Autodesk Inventor part; units mm, degrees
ref_plane "YZ Plane" through (0, 0, 0) normal (1, 0, 0) x (0, 1, 0)
ref_plane "XZ Plane" through (0, 0, 0) normal (0, 1, 0) x (-1, 0, 0)
ref_plane "XY Plane" through (0, 0, 0) normal (0, 0, 1) x (1, 0, 0)
sketch "Sketch1" plane through (0, 0, 0) normal (0, 1, 0) x (-1, 0, 0)
  circle A0 centre (0, 0) radius 30.734
  line L0 (-20.32, 68.58) -> (350.52, 68.58)
  line L1 (381, 38.1) -> (381, -38.1)
  line L2 (350.52, -68.58) -> (-20.32, -68.58)
  line L3 (-50.8, -38.1) -> (-50.8, 38.1)
  arc A1 (-20.32, 68.58) -> (-50.8, 38.1) centre (-20.32, 38.1) ccw
  arc A2 (-50.8, -38.1) -> (-20.32, -68.58) centre (-20.32, -38.1) ccw
  arc A3 (381, 38.1) -> (350.52, 68.58) centre (350.52, 38.1) ccw
  arc A4 (350.52, -68.58) -> (381, -38.1) centre (350.52, -38.1) ccw
  point P0 (-50.8, 68.58)
  point P1 (381, -68.58)
  point P2 (-50.8, -68.58)
  dimension "d0" = 61.468
  dimension "d1" = 137.16
  dimension "d2" = 431.8
  dimension "d3" = 50.8
  dimension "d4" = 68.58
  dimension "d5" = 30.48
extrude "Extrusion1" add sketch "Sketch1" against normal blind 129.54
sketch "Sketch2" plane through (0, -129.54, 0) normal (0, -1, 0) x (1, 0, 0)
  circle A0 centre (0, 0) radius 38.1
  dimension "d17" = 76.2
extrude "Extrusion2" add sketch "Sketch2" against normal blind 93.98
sketch "Sketch3" plane through (0, 0, 0) normal (0, 1, 0) x (1, 0, 0)
  line L0 (50.8, 38.1) -> (50.8, -38.1)
  line L1 (50.8, 0) -> (-132.08, 0)
  line L2 (20.32, -68.58) -> (-350.52, -68.58)
  line L3 (-132.08, -68.58) -> (-434.975, -68.58)
  line L4 (-434.975, -68.58) -> (-434.975, 68.58)
  line L5 (-434.975, 68.58) -> (-132.08, 68.58)
  line L6 (-132.08, 68.58) -> (-132.08, -68.58)
  point P0 (0, 0)
  dimension "d10" = 182.88
extrude "Extrusion3" cut sketch "Sketch3" against normal blind 35.2425
sketch "Sketch4" plane through (0, -35.2425, 0) normal (0, 1, 0) x (1, 0, 0)
  line L0 (-381, -38.1) -> (-381, 38.1)
  line L1 (-381, 0) -> (-328.6125, 0)
  line L2 (-381, 0) -> (-317.5, 0)
  circle A0 centre (-317.5, 0) radius 30.48
  point P0 (0, 0)
  dimension "d14" = 60.96
  dimension "d18" = 317.5
extrude "Extrusion4" add sketch "Sketch4" along normal blind 35.56
properties part number "Shoulder2 Link"
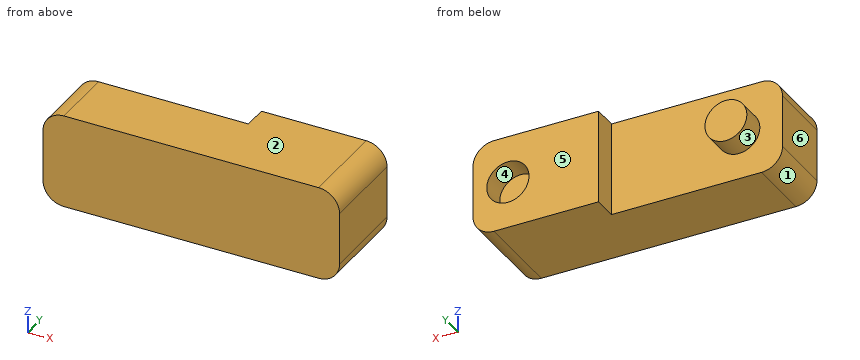
Read the model definition and answer for the solid it produces. Units are mm, in the model's axes. Face numbers are marked on the shaded views. A direction names the side the tool comes from. Give positions to 0.01 mm unless a question says otherwise; leave off trailing zeros. Write each loop counter-clockwise with the first axis right and the second up, starting at its lowest first coordinate (ties: lowest second). Pieces come first, ordered by that corner, then holes. Notation, with made-up numbers: (89.25, 68.25) -> (102.25, 68.25) arc R25 cw to (102.25, 95.25) -> close; hole circle Ø1 at (54.25, 50). An arc over 180 degrees is marked (long way). Answer as a JSON object with one key per item and string values. Group by question number.
1) Find section B-B (x = 0). Write down the section's boundary in (y, z).
2) A tool of negligible diameter and unlimited length cuts with its end or side. For the marked faces 4, 5 and 6, from which of +Z, -Z, +X, -X, +Y, -Y can it reach the whole face along a straight path? Write none if from no direction.
3) Consider L1, parallel to Z at x = 0, y = -15; L2, parallel to Y at x = -339.5, z = -55.5; L3, parallel to Y at x = -37, z = 47.5. Determine where each line is inside the solid, lowest interval first. Write a range as from..to.
4) Find section C-C (x = -317.5). Write down the section's boundary in (y, z).
5) Find section A-A (z = 0). Write down the section's boundary in (x, y).
6) The mould has two halves that part along X. Classify the marked faces 1, 2 and 3: +X half, -X half, draft (parallel to the pull), parting line (faces both ways), or undercut.
7) Find section D-D (z = -48). Write down the section's boundary in (x, y).
8) Each of these flat-tipped pins is pushed along its axis until it touches: P1, Ø4, axis at y = -23.5, z = 44.5, coming from the +X side; P2, Ø10, axis at x = -283, z = 23, coming from the +Y side; P3, Ø3, axis at y = -31, z = -26, coming from the -X side. Where does it stop, or does it pass through?
Values follow:
{
 "1": {"outline": "(-129.54, -68.58) -> (0, -68.58) -> (0, -30.73) -> (-35.56, -30.73) -> (-35.56, 30.73) -> (0, 30.73) -> (0, 68.58) -> (-129.54, 68.58) -> close"},
 "2": {"face 4": "+Y", "face 5": "+Z, -Z, +X, +Y", "face 6": "+Z, -Z, -X, +Y, -Y"},
 "3": {"L1": "z = -68.58..-30.73, 30.73..68.58", "L2": "y = -129.54..-35.24", "L3": "y = -129.54..0"},
 "4": {"outline": "(-129.54, -68.58) -> (-35.24, -68.58) -> (-35.24, -30.48) -> (0.32, -30.48) -> (0.32, 30.48) -> (-35.24, 30.48) -> (-35.24, 68.58) -> (-129.54, 68.58) -> close"},
 "5": {"outline": "(-381, -129.54) -> (50.8, -129.54) -> (50.8, 0) -> (30.73, 0) -> (30.73, -35.56) -> (-30.73, -35.56) -> (-30.73, 0) -> (-132.08, 0) -> (-132.08, -35.24) -> (-287.02, -35.24) -> (-287.02, 0.32) -> (-347.98, 0.32) -> (-347.98, -35.24) -> (-381, -35.24) -> close"},
 "6": {"face 1": "-X half", "face 2": "draft", "face 3": "undercut"},
 "7": {"outline": "(-379.35, -129.54) -> (49.15, -129.54) -> (49.15, 0) -> (-132.08, 0) -> (-132.08, -35.24) -> (-379.35, -35.24) -> close"},
 "8": {"P1": "stops at x = 50.48", "P2": "stops at y = -35.24", "P3": "stops at x = -335.63"}
}
